For this review, use the dimensioned drawing (mm, ordinates from the lowest corner) and the shaded views. A direction names the side the tool comes from. Give positions to 0.01 mm unless a question says otherwise; leave off trailing zeros. Write each loop counter-clockwise with the first axis right and the second up, starting at its lowest first coordinate (ties: lowest second). Pieces come first, ordered by that corner, then holes. Notation, with made-up numbers: (56.25, 69) - (88.25, 69) arc R25 ccw to (88.25, 107) - close; hole circle Ø10 at (42, 61). An arc over 180 degrees is marked (long way). Use a Markdown table: item, result. Add a question column.
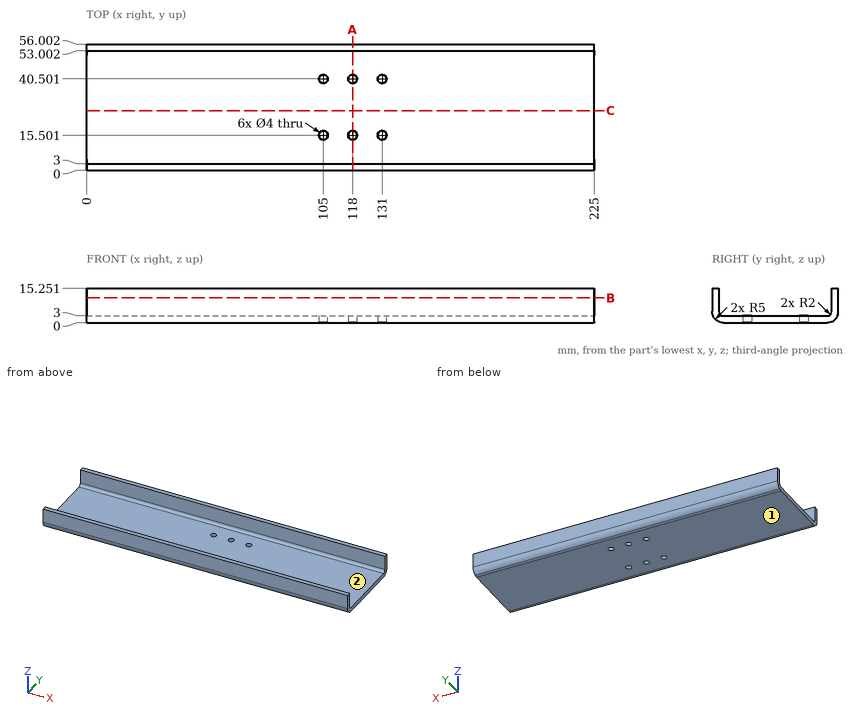
(1) Insertion check: pin 1 (5 mm diameter, centred on x = 118, y = 40.5, fed in from +Z); pin 2 (5 mm diameter, centred on x = 105, y = 40.5, fed in from -Z); pin 3 (3.5 mm diameter, centred on x = 105, y = 15.5, fed in from -Z). Each pin has a flat end and moves straight along its axis. Give the tip position at first contact, or say it passes through.
(2) Add section A-A (x = 118). State the section outline as (y, z) points.
(3) For line 1 along Y through (x, z) = (103, 13); line 2 along Y through (x, z) = (131, 2.2) (1 decimal); line 3 along Y through (x, z) = (118, 2.45), list the stretches that pass through material, from the lowest coordinate up.
(4) Add section B-B (z = 11). State the section outline as (x, y) points.
(5) Tool access review of the marked faces 1 and 2: name each direction out of +Z, -Z, +X, -X, +Y, -Y from which nothing blocks a thin tool from reaching the whole face with its end or side.
(6) Add section C-C (y = 26.5). State the section outline as (x, z) points, and give its area (3 significant figures).
Answers follow:
| question | item | result |
|---|---|---|
| 1 | pin 1 | z = 3 |
| 1 | pin 2 | z = 0 |
| 1 | pin 3 | through |
| 2 | outline | (0, 5) arc R5 ccw to (5, 0) - (13.5, 0) - (13.5, 3) - (5, 3) arc R2 cw to (3, 5) - (3, 15.25) - (0, 15.25) - close; (17.5, 0) - (38.5, 0) - (38.5, 3) - (17.5, 3) - close; (42.5, 0) - (51, 0) arc R5 ccw to (56, 5) - (56, 15.25) - (53, 15.25) - (53, 5) arc R2 cw to (51, 3) - (42.5, 3) - close |
| 3 | line 1 | 0 to 3, 53 to 56 |
| 3 | line 2 | 0.9 to 13.5, 17.5 to 38.5, 42.5 to 55.1 |
| 3 | line 3 | 0.7 to 13.5, 17.5 to 38.5, 42.5 to 55.3 |
| 4 | outline | (0, 0) - (225, 0) - (225, 3) - (0, 3) - close; (0, 53) - (225, 53) - (225, 56) - (0, 56) - close |
| 5 | face 1 | -Z, +X, -X, +Y, -Y |
| 5 | face 2 | +Z, +X, -X |
| 6 | outline | (0, 0) - (225, 0) - (225, 3) - (0, 3) - close |
| 6 | area | 675 mm^2 |
